Check sheet for the modelled part. Datum: model origin and axes. Units: mm. A direction names the side the tool comes from. Round coordinates to 2 decimals unless told otherwise and drop trailing zeros. Order: outer loops, then holes, each group sorted by start corner. A loop starts at its lowest first (then second) coordinate and runs counter-clockwise, first axis right, second up.
```python
from build123d import *

# Parameters (mm, degrees)
F0_R     = 17.78
F0_W     = 50.8
F0_H     = 38.1
F0_R_2   = 7.62
F1_DEPTH = 10.414
F2_DEPTH = 1.27
F3_R     = 5.08


with BuildPart() as f1:
    # F0 (on Top) → F1 (new body)
    with BuildSketch(Plane.XY):
        with BuildLine():
            Line((25.4, 52.07), (-25.4, 52.07))
            ThreePointArc((-25.4, 52.07), (-28.9921024484, 50.5821024484), (-30.48, 46.99))
            Line((-30.48, 46.99), (-30.48, -46.99))
            ThreePointArc((-30.48, -46.99), (-28.9921024484, -50.5821024484), (-25.4, -52.07))
            Line((-25.4, -52.07), (25.4, -52.07))
            ThreePointArc((25.4, -52.07), (28.9921024484, -50.5821024484), (30.48, -46.99))
            Line((30.48, -46.99), (30.48, 46.99))
            ThreePointArc((30.48, 46.99), (28.9921024484, 50.5821024484), (25.4, 52.07))
        make_face()
        with Locations((0, -21.59)):
            Circle(F0_R, mode=Mode.SUBTRACT)
        with Locations((0, 26.67)):
            Rectangle(F0_W, F0_H, mode=Mode.SUBTRACT)
        with Locations((0, 26.67)):
            Rectangle(F0_W, F0_H)
        with Locations((0, -21.59)):
            Circle(F0_R)
        with Locations((0, -21.59)):
            Circle(F0_R_2, mode=Mode.SUBTRACT)
        with Locations((0, -21.59)):
            Circle(F0_R_2)
    extrude(amount=F1_DEPTH)

    # F0 (on Top) → F2 (join)
    with BuildSketch(Plane.XY):
        with Locations((0, -21.59)):
            Circle(F0_R)
        with Locations((0, -21.59)):
            Circle(F0_R_2, mode=Mode.SUBTRACT)
        with Locations((0, 26.67)):
            Rectangle(F0_W, F0_H)
    extrude(amount=-F2_DEPTH)

    # F3
    f3_edges = [f1.edges().sort_by_distance(p)[0] for p in [
        (0, -52.07, 10.414),
        (0, 52.07, 10.414),
    ]]
    fillet(f3_edges, radius=F3_R)


solid = f1.part
```
Item 1: Scan lines: line 1 along Y through (x, z) = (0, -0.75); line 2 along Z through (x, y) = (8.5, 46); line 3 along Y through (x, z) = (5.5, -0.25). Record each from-to range of solid material in increasing order.
Answer:
line 1: y = -39.37 to -29.21, -13.97 to -3.81, 7.62 to 45.72
line 2: z = 0 to 10.41
line 3: y = -38.5 to -26.86, -16.32 to -4.68, 7.62 to 45.72
Item 2: Sectioned sample at A-A (y = -21.59). Record the cut outline in (x, z), and give its area (3 significant figures).
Answer:
outline: (-30.48, 0) - (-17.78, 0) - (-17.78, -1.27) - (-7.62, -1.27) - (-7.62, 0) - (7.62, 0) - (7.62, -1.27) - (17.78, -1.27) - (17.78, 0) - (30.48, 0) - (30.48, 5.33) arc R5.08 ccw to (25.4, 10.41) - (-25.4, 10.41) arc R5.08 ccw to (-30.48, 5.33) - close
area: 650 mm2
Item 3: Sectioned sample at B-B (x = -22). Record the cut outline in (y, z), and give its area (3 significant figures).
Answer:
outline: (-52.07, 0) - (7.62, 0) - (7.62, -1.27) - (45.72, -1.27) - (45.72, 0) - (52.07, 0) - (52.07, 5.33) arc R5.08 ccw to (46.99, 10.41) - (-46.99, 10.41) arc R5.08 ccw to (-52.07, 5.33) - close
area: 1,120 mm2
Item 4: Go/stop test with flat-tipped pins: P1, Ø0.6, axis at y = 27, z = -0.5, coming from the +X side; P2, Ø0.6, axis at y = 33.5, z = -0.5, coming from the -X side; P3, Ø7.5, axis at x = -2, y = -22, coming from the -Z side. Record where each tip stops, or that it passes through.
Answer:
P1: stops at x = 25.4
P2: stops at x = -25.4
P3: stops at z = 0
Item 5: Access from +Z, -Z, +X, -X, +Y, -Y to the whole of each face (thin tool, end or side, straight path). Record for faces 5 (the flat face through (0, -52.07, 3)), 6 (the cylindrical face through (-0.992, -14.035, -0.626)).
Answer:
face 5: +Z, -Z, +X, -X, -Y
face 6: -Z
Item 6: Release check for a two-part mould opening along Y. For faces 1 (the cylindrical face through (9.56, -6.6, -0.63)), 2 (the cylindrical face through (29.031, 50.542, 2.63)), 3 (the cylindrical face through (28.95, 0.66, 8.97)), 4 (the flat face through (0, -21, 0)) record: released by +Y, released by -Y, zero draft, split by the parting line, or undercut.
Answer:
face 1: undercut
face 2: released by +Y
face 3: zero draft
face 4: undercut
Item 7: Sectioned sample at D-D (y = 37.5). Record the cut outline in (x, z).
Answer:
outline: (-30.48, 0) - (-25.4, 0) - (-25.4, -1.27) - (25.4, -1.27) - (25.4, 0) - (30.48, 0) - (30.48, 5.33) arc R5.08 ccw to (25.4, 10.41) - (-25.4, 10.41) arc R5.08 ccw to (-30.48, 5.33) - close
Item 8: Sectioned sample at C-C (z = 7). Record the cut outline in (x, y), and give its area (3 significant figures).
Answer:
outline: (-30.2, -46.99) arc R4.8 ccw to (-25.4, -51.79) - (25.4, -51.79) arc R4.8 ccw to (30.2, -46.99) - (30.2, 46.99) arc R4.8 ccw to (25.4, 51.79) - (-25.4, 51.79) arc R4.8 ccw to (-30.2, 46.99) - close
area: 6,240 mm2
